Source: CAD feature listing. Evaluate the final solid. Frame: model axes, mm. A direction names the side the tool comes from. Give positions to 0.01 mm unless a question says otherwise; leave off trailing zeros. Write each loop counter-clockwise with the first axis right and the second up, starting at its lowest first coordinate (ties: lowest second). Pieces come first, ordered by that corner, then holes. Notation, with made-up numbers: (83.5, -23.75) -> (112.5, -23.75) arc R25 ccw to (112.5, 8.25) -> close; hole circle Ø8 at (-30, 82). An arc over 180 degrees is marked (long way). Write item = value, one per line.
from build123d import *

# Parameters (mm, degrees)
CROQUIS1_R              = 3.975
CROQUIS1_R_2            = 1.5
SALIENTE_EXTRUIR1_DEPTH = 10.2


with BuildPart() as part:
    # Croquis1 → Saliente-Extruir1 (new body)
    with BuildSketch(Plane(origin=(0, 0, 0), x_dir=(1, 0, 0), z_dir=(0, 1, 0))):
        with BuildLine():
            Line((-34.10243875, 6.486534721), (-15.364079564, 6.486534721))
            Line((-15.364079564, 6.486534721), (-15.364079564, 23.436691068))
            ThreePointArc((-15.364079564, 23.436691068), (-5.364079564, 33.436691068), (4.635920436, 23.436691068))
            Line((4.635920436, 23.436691068), (4.635920436, 6.486534721))
            Line((4.635920436, 6.486534721), (23.768585867, 6.486534721))
            ThreePointArc((23.768585867, 6.486534721), (24.318891967, 6.08655714), (24.635920436, 5.484633707))
            Line((24.635920436, 5.484633707), (24.635920436, -6.563308932))
            Line((24.635920436, -6.563308932), (-35.364079564, -6.563308932))
            Line((-35.364079564, -6.563308932), (-35.364079564, 5.386400848))
            ThreePointArc((-35.364079564, 5.386400848), (-34.900990267, 6.128822933), (-34.10243875, 6.486534721))
        make_face()
        with Locations(Location((-5.364079564, 23.436691068, 0), (0, 0, 270))):
            Circle(CROQUIS1_R, mode=Mode.SUBTRACT)
        with Locations(Location((-24.733259157, 3.398021726, 0), (0, 0, 270))):
            Circle(CROQUIS1_R_2, mode=Mode.SUBTRACT)
        with Locations(Location((14.202253152, 3.398021726, 0), (0, 0, 270))):
            Circle(CROQUIS1_R_2, mode=Mode.SUBTRACT)
    extrude(amount=SALIENTE_EXTRUIR1_DEPTH)


solid = part.part
(1) Section query D-D (x = 19.5). Return loops of the section in (y, z).
Values follow:
outline = (0, -6.49) -> (10.2, -6.49) -> (10.2, 6.56) -> (0, 6.56) -> close
(2) First-contact query: pin 1 (4 mm diameter, centred on x = -19, y = 7.5, fed in from -Z); pin 2 (1.8 mm diameter, centred on x = -24.73, z = -3.4, fed in from -Y); pin 3 (4 mm diameter, centred on y = 7.5, z = -25.5, fed in from -X). Flat tips, straight axial feed; report the tip coordinate or a pass-through.
Values follow:
pin_1 = -6.49
pin_2 = through
pin_3 = -15.36
(3) Access query for faces 4 (the face through (-15.364, 5, -15)), 5 (the face through (-23.719, 5.029, -4.504)), 6 (the face through (4.636, 5, -15)). Directions: +Z, -Z, +X, -X, +Y, -Y. A direction counts if a zero-diameter tool reaches every point of the face in a straight line with its end or side. Return the directions, or none.
Values follow:
face_4 = -Z, -X, +Y, -Y
face_5 = +Y, -Y
face_6 = -Z, +X, +Y, -Y
(4) Section query C-C (x = -6). Return loops of the section in (y, z).
Values follow:
outline = (0, -33.42) -> (10.2, -33.42) -> (10.2, -27.36) -> (0, -27.36) -> close; (0, -19.51) -> (10.2, -19.51) -> (10.2, 6.56) -> (0, 6.56) -> close
(5) Section query B-B (z = -25.5). Return loops of the section in (x, y), plus the area to 3 significant figures.
Values follow:
outline = (-15.15, 0) -> (-8.76, 0) -> (-8.76, 10.2) -> (-15.15, 10.2) -> close; (-1.97, 0) -> (4.42, 0) -> (4.42, 10.2) -> (-1.97, 10.2) -> close
area = 130 mm2
(6) Pull-direction query (Z, two-part tool) for faces 1 (the face through (14, 5, -6.487)), 2 (the face through (-5.189, 5.029, -27.408)), 3 (the face through (24.636, 5, 0)); classes: pulls with the +Z half, pulls with the -Z half, needs draft (parallel to the pull), parting line crosses it, or undercut.
Values follow:
face_1 = pulls with the -Z half
face_2 = undercut
face_3 = needs draft
(7) Section query A-A (y = 5.75). Return loops of the section in (x, z) (3 decimals), plus the area to 3 significant figures.
Values follow:
outline = (-35.364, -5.386) arc R1.5 ccw to (-34.102, -6.487) -> (-15.364, -6.487) -> (-15.364, -23.437) arc R10 ccw to (4.636, -23.437) -> (4.636, -6.487) -> (23.769, -6.487) arc R1.5 ccw to (24.636, -5.485) -> (24.636, 6.563) -> (-35.364, 6.563) -> close; hole circle Ø3 at (-24.733, -3.398); hole circle Ø7.95 at (-5.364, -23.437); hole circle Ø3 at (14.202, -3.398)
area = 1,210 mm2
(8) Material intervals for line 1 (Z direction, x = 10, y = 3.5); line 2 (X direction, y = 9.25, z = -14); line 3 (Z direction, x = -2, y = 5), sorted ascending.
Values follow:
line_1 = -6.49 to 6.56
line_2 = -15.36 to 4.64
line_3 = -32.85 to -25.55, -21.32 to 6.56
